Can you work these out from the model? Positions are in its coordinate system, mm. Give positions to 0.01 mm unless a question says otherwise; leave off trailing zeros. Loops run counter-clockwise (first coordinate to the right, second up) from the corner with the lowest first, then second, coordinate; pieces in that order, holes last. Notation, with made-up numbers: (-32.75, 20) -> (23.25, 20) arc R14 ccw to (23.25, 41) -> close; hole circle Ø8 at (64, -9). An arc over 180 degrees is marked (long way). Use CSV: the item, a comma, the result in double quotes.
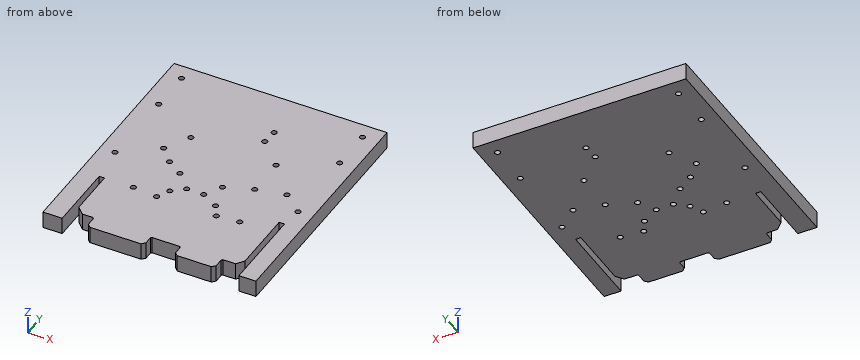
from build123d import *

# Parameters (mm, degrees)
BOARD_OUTLINE_DEPTH = 0.8
SKETCH2_R           = 0.127
NPTH_DEPTH          = 16.260733927


with BuildPart() as part:
    # Sketch1 → Board_Outline (new body)
    with BuildSketch(Plane.XY):
        Polygon((10, 0), (10, 11.5), (0, 11.5), (0, 0), (0.9, 0), (0.9, 3.25), (1.15, 3.25), (1.15, 1), (1.5, 0.65), (2, 0.65), (2.05, 0.6), (2.05, 0.15), (2.2, 0), (4.6, 0), (4.75, 0.15), (4.75, 0.55), (4.8, 0.6), (6.1, 0.6), (6.15, 0.55), (6.15, 0.15), (6.3, 0), (7.9, 0), (8.05, 0.15), (8.05, 0.6), (8.1, 0.65), (8.7, 0.65), (8.95, 1), (8.95, 4), (9.2, 4), (9.2, 0), align=None)
    extrude(amount=BOARD_OUTLINE_DEPTH)

    # Sketch2 → NPTH (cut, through all)
    with BuildSketch(Plane.XY):
        with Locations((4.5, 4.2)):
            Circle(SKETCH2_R)
        with Locations((5.875, 9.3)):
            Circle(SKETCH2_R)
        with Locations((5.3, 4.2)):
            Circle(SKETCH2_R)
        with Locations((5.825, 8.575)):
            Circle(SKETCH2_R)
        with Locations((7.5, 3.25)):
            Circle(SKETCH2_R)
        with Locations((2.5, 3.25)):
            Circle(SKETCH2_R)
        with Locations((3.75, 5)):
            Circle(SKETCH2_R)
        with Locations((5.75, 5)):
            Circle(SKETCH2_R)
        with Locations((7, 5.5)):
            Circle(SKETCH2_R)
        with Locations((3, 5.5)):
            Circle(SKETCH2_R)
        with Locations((3, 7.375)):
            Circle(SKETCH2_R)
        with Locations((7, 7.375)):
            Circle(SKETCH2_R)
        with Locations((9.25, 8.75)):
            Circle(SKETCH2_R)
        with Locations((0.75, 8.75)):
            Circle(SKETCH2_R)
        with Locations((9.25, 10.75)):
            Circle(SKETCH2_R)
        with Locations((0.75, 10.75)):
            Circle(SKETCH2_R)
        with Locations((9.3, 5)):
            Circle(SKETCH2_R)
        with Locations((0.7, 5)):
            Circle(SKETCH2_R)
        with Locations((3.95, 3.75)):
            Circle(SKETCH2_R)
        with Locations((8.35, 5.8)):
            Circle(SKETCH2_R)
        with Locations((6.1, 3.75)):
            Circle(SKETCH2_R)
        with Locations((3.65, 3.15)):
            Circle(SKETCH2_R)
        with Locations((6.45, 3.15)):
            Circle(SKETCH2_R)
        with Locations((2.35, 6.2)):
            Circle(SKETCH2_R)
    extrude(amount=NPTH_DEPTH, mode=Mode.SUBTRACT)


solid = part.part
(1) If we section it at D-D, the plane x = 7.5: Write out the boundary of the cut face in (y, z), then the cut area to 3 significant figures.
Answer sheet:
outline,"(0, 0) -> (3.12, 0) -> (3.12, 0.8) -> (0, 0.8) -> close; (3.38, 0) -> (11.5, 0) -> (11.5, 0.8) -> (3.38, 0.8) -> close"
area,"9.00 mm2"
(2) If I drill on L1, parallel to X at y = 3.75, z = 0.6; L2, parallel to X at y = 1.75, z = 0.5; L3, parallel to X at y = 10.75, z = 0.65, over which ranges is the centre line in solid material (lowest first)? Write a range as from..to.
Answer sheet:
L1,"x = 0..3.82, 4.08..5.97, 6.23..8.95, 9.2..10"
L2,"x = 0..0.9, 1.15..8.95, 9.2..10"
L3,"x = 0..0.62, 0.88..9.12, 9.38..10"
(3) If we section it at B-B, the plane y = 6.2: Write out the boundary of the cut face in (x, z), then the cut area to 3 significant figures.
Answer sheet:
outline,"(0, 0) -> (2.22, 0) -> (2.22, 0.8) -> (0, 0.8) -> close; (2.48, 0) -> (10, 0) -> (10, 0.8) -> (2.48, 0.8) -> close"
area,"7.80 mm2"
(4) If we section it at A-A, the plane y = 3.75: Write out the boundary of the cut face in (x, z), then the cut area to 3 significant figures.
Answer sheet:
outline,"(0, 0) -> (3.82, 0) -> (3.82, 0.8) -> (0, 0.8) -> close; (4.08, 0) -> (5.97, 0) -> (5.97, 0.8) -> (4.08, 0.8) -> close; (6.23, 0) -> (8.95, 0) -> (8.95, 0.8) -> (6.23, 0.8) -> close; (9.2, 0) -> (10, 0) -> (10, 0.8) -> (9.2, 0.8) -> close"
area,"7.39 mm2"
(5) If we section it at C-C, the plane x = 3: Write out the boundary of the cut face in (y, z), then the cut area to 3 significant figures.
Answer sheet:
outline,"(0, 0) -> (5.37, 0) -> (5.37, 0.8) -> (0, 0.8) -> close; (5.63, 0) -> (7.25, 0) -> (7.25, 0.8) -> (5.63, 0.8) -> close; (7.5, 0) -> (11.5, 0) -> (11.5, 0.8) -> (7.5, 0.8) -> close"
area,"8.79 mm2"
